from build123d import *

# Parameters (mm, degrees)
SKETCH_1_R               = 23.15
EXTRUDE_1_DEPTH          = 19
SKETCH_2_R               = 3.3
CUT_EXTRUDE_1_DEPTH      = 1
CUT_EXTRUDE_1_DEPTH_BACK = 20
PATTERN_CIRCULAR_1_COUNT = 4
FILLET_1_R               = 1
SKETCH_6_R               = 23.65
EXTRUDE_2_DEPTH          = 0.5
SKETCH_7_R               = 23.65
SKETCH_7_R_2             = 23.15
EXTRUDE_1_2_DEPTH        = 3.5
EXTRUDE_5_DEPTH          = 6
PATTERN_CIRCULAR_3_COUNT = 8
SKETCH_18_R              = 3.3
CUT_EXTRUDE_2_DEPTH      = 7.5
SKETCH_19_R              = 6.3
SKETCH_19_R_2            = 3.3
EXTRUDE_6_DEPTH          = 4
CHAMFER_1_SIZE           = 1
FILLET_3_R               = 0.5
FILLET_4_R               = 0.5


with BuildPart() as part:
    # Sketch 1 → Extrude 1 (new body)
    with BuildSketch(Plane(origin=(0, 0, 0), x_dir=(1, 0, 0), z_dir=(0, 1, 0))):
        Circle(SKETCH_1_R)
    extrude(amount=EXTRUDE_1_DEPTH)

    # Sketch 5 → Hole Wizard M3 _1 (revolve, cut)
    with BuildSketch(Plane(origin=(-12, 19, 0), x_dir=(0, 0, 1), z_dir=(1, 0, 0))):
        Polygon((0, 0), (0, 4.751075774), (1.25, 4), (1.25, 0), align=None)
    hole_wizard_m3_1 = revolve(axis=Axis((-12, 25.35, 0), (0, -1, 0)), mode=Mode.SUBTRACT)

    # Sketch 2 → Cut-Extrude 1 (cut, two sides)
    with BuildSketch(Plane(origin=(0, 19, 0), x_dir=(1, 0, 0), z_dir=(0, 1, 0))) as cut_extrude_1_sk:
        Circle(SKETCH_2_R)
    extrude(amount=CUT_EXTRUDE_1_DEPTH, mode=Mode.SUBTRACT)
    extrude(cut_extrude_1_sk.sketch, amount=-CUT_EXTRUDE_1_DEPTH_BACK, mode=Mode.SUBTRACT)

    # Pattern Circular 1: Hole Wizard M3 _1 ×4 about axis
    pattern_circular_1_axis = Axis((0, 0, 0), (0, 1, 0))
    for i in range(1, PATTERN_CIRCULAR_1_COUNT):
        add(hole_wizard_m3_1.rotate(pattern_circular_1_axis, i * 360 / PATTERN_CIRCULAR_1_COUNT), mode=Mode.SUBTRACT)

    # Fillet 1
    fillet_1_edges = [part.edges().sort_by_distance(p)[0] for p in [
        (-23.15, 19, 0),
    ]]
    fillet(fillet_1_edges, radius=FILLET_1_R)

    # Sketch 6 → Extrude 2 (add)
    with BuildSketch(Plane.XZ):
        Circle(SKETCH_6_R)
    extrude(amount=EXTRUDE_2_DEPTH)

    # Sketch 7 → Extrude 1 2 (add)
    with BuildSketch(Plane.XZ.offset(0.5)):
        Circle(SKETCH_7_R)
        Circle(SKETCH_7_R_2, mode=Mode.SUBTRACT)
    extrude(amount=EXTRUDE_1_2_DEPTH)

    # Sketch 8 → Extrude 5 (add)
    with BuildSketch(Plane.XZ.offset(0.5)):
        with BuildLine():
            Line((-21.839675903, 3.694733612), (-22.825665785, 3.861538741))
            ThreePointArc((-22.825665785, 3.861538741), (-23.15, 0), (-22.825665785, -3.861538741))
            Line((-22.825665785, -3.861538741), (-21.839675903, -3.694733612))
            ThreePointArc((-21.839675903, -3.694733612), (-20.969056247, -2.594652523), (-19.772134146, -1.862850316))
            ThreePointArc((-19.772134146, -1.862850316), (-18.5, 0), (-19.772134146, 1.862850316))
            ThreePointArc((-19.772134146, 1.862850316), (-20.969056247, 2.594652523), (-21.839675903, 3.694733612))
        make_face()
        with BuildLine():
            ThreePointArc((-13.409662832, 18.870703292), (-16.369521984, 16.369521984), (-18.870703292, 13.409662832))
            Line((-18.870703292, 13.409662832), (-18.055554121, 12.830411738))
            ThreePointArc((-18.055554121, 12.830411738), (-16.662058262, 12.992665473), (-15.298244224, 12.663776043))
            ThreePointArc((-15.298244224, 12.663776043), (-13.081475452, 13.081475452), (-12.663776043, 15.298244224))
            ThreePointArc((-12.663776043, 15.298244224), (-12.992665473, 16.662058262), (-12.830411738, 18.055554121))
            Line((-12.830411738, 18.055554121), (-13.409662832, 18.870703292))
        make_face()
        with BuildLine():
            Line((-18.055554121, -12.830411738), (-18.870703292, -13.409662832))
            ThreePointArc((-18.870703292, -13.409662832), (-16.369521984, -16.369521984), (-13.409662832, -18.870703292))
            Line((-13.409662832, -18.870703292), (-12.830411738, -18.055554121))
            ThreePointArc((-12.830411738, -18.055554121), (-12.992665473, -16.662058261), (-12.663776043, -15.298244224))
            ThreePointArc((-12.663776043, -15.298244224), (-13.081475452, -13.081475452), (-15.298244224, -12.663776043))
            ThreePointArc((-15.298244224, -12.663776043), (-16.662058261, -12.992665473), (-18.055554121, -12.830411738))
        make_face()
        with BuildLine():
            ThreePointArc((18.870703292, 13.409662832), (16.369521984, 16.369521984), (13.409662832, 18.870703292))
            Line((13.409662832, 18.870703292), (12.830411738, 18.055554121))
            ThreePointArc((12.830411738, 18.055554121), (12.992665473, 16.662058262), (12.663776043, 15.298244224))
            ThreePointArc((12.663776043, 15.298244224), (13.081475452, 13.081475452), (15.298244224, 12.663776043))
            ThreePointArc((15.298244224, 12.663776043), (16.662058261, 12.992665473), (18.055554121, 12.830411738))
            Line((18.055554121, 12.830411738), (18.870703292, 13.409662832))
        make_face()
        with BuildLine():
            Line((12.830411738, -18.055554121), (13.409662832, -18.870703292))
            ThreePointArc((13.409662832, -18.870703292), (16.369521984, -16.369521984), (18.870703292, -13.409662832))
            Line((18.870703292, -13.409662832), (18.055554121, -12.830411738))
            ThreePointArc((18.055554121, -12.830411738), (16.662058262, -12.992665473), (15.298244224, -12.663776043))
            ThreePointArc((15.298244224, -12.663776043), (13.081475452, -13.081475452), (12.663776043, -15.298244224))
            ThreePointArc((12.663776043, -15.298244224), (12.992665473, -16.662058261), (12.830411738, -18.055554121))
        make_face()
        with BuildLine():
            ThreePointArc((22.825665785, -3.861538741), (23.15, 0), (22.825665785, 3.861538741))
            Line((22.825665785, 3.861538741), (21.839675903, 3.694733612))
            ThreePointArc((21.839675903, 3.694733612), (20.969056247, 2.594652523), (19.772134146, 1.862850316))
            ThreePointArc((19.772134146, 1.862850316), (18.5, 0), (19.772134146, -1.862850316))
            ThreePointArc((19.772134146, -1.862850316), (20.969056247, -2.594652523), (21.839675903, -3.694733612))
            Line((21.839675903, -3.694733612), (22.825665785, -3.861538741))
        make_face()
    extrude(amount=EXTRUDE_5_DEPTH)

    # Sketch 17 → Hole Wizard M2 _1 (revolve, cut)
    with BuildSketch(Plane(origin=(-20.5, -6.5, 0), x_dir=(0, 0, -1), z_dir=(1, 0, 0))):
        Polygon((0, 0), (0, 5.680688495), (0.8, 5.2), (0.8, 0), align=None)
    hole_wizard_m2_1 = revolve(axis=Axis((-20.5, -12.85, 0), (0, 1, 0)), mode=Mode.SUBTRACT)

    # Pattern Circular 3: Hole Wizard M2 _1 ×8 about axis, 1 skipped
    pattern_circular_3_axis = Axis((0, 0, 0), (0, 1, 0))
    add([hole_wizard_m2_1.rotate(pattern_circular_3_axis, i * 360 / PATTERN_CIRCULAR_3_COUNT) for i in range(1, PATTERN_CIRCULAR_3_COUNT) if i not in (2,)], mode=Mode.SUBTRACT)

    # Sketch 18 → Cut-Extrude 2 (cut, through all)
    with BuildSketch(Plane(origin=(0, 0, 0), x_dir=(1, 0, 0), z_dir=(0, 1, 0))):
        Circle(SKETCH_18_R)
    extrude(amount=-CUT_EXTRUDE_2_DEPTH, mode=Mode.SUBTRACT)

    # Sketch 19 → Extrude 6 (add)
    with BuildSketch(Plane.XZ.offset(0.5)):
        Circle(SKETCH_19_R)
        Circle(SKETCH_19_R_2, mode=Mode.SUBTRACT)
    extrude(amount=EXTRUDE_6_DEPTH)

    # Chamfer 1
    chamfer_1_edges = [part.edges().sort_by_distance(p)[0] for p in [
        (-3.3, 19, 0),
    ]]
    chamfer(chamfer_1_edges, length=CHAMFER_1_SIZE)

    # Fillet 3
    fillet_3_edges = [part.edges().sort_by_distance(p)[0] for p in [
        (-6.3, -4.5, 0),
    ]]
    fillet(fillet_3_edges, radius=FILLET_3_R)

    # Fillet 4
    fillet_4_edges = [part.edges().sort_by_distance(p)[0] for p in [
        (-3.3, -4.5, 0),
    ]]
    fillet(fillet_4_edges, radius=FILLET_4_R)


solid = part.part
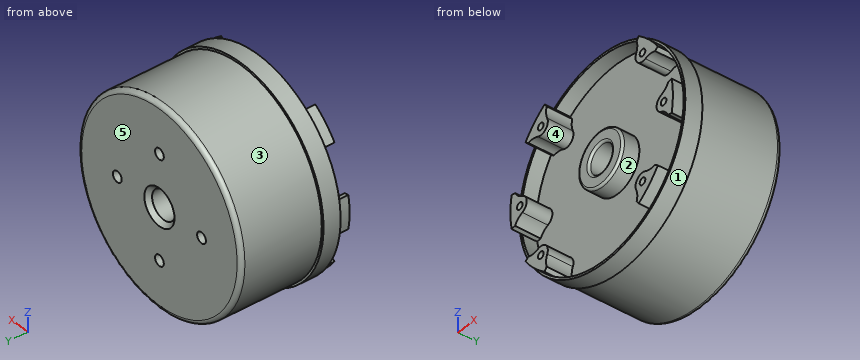
CAD build for the part. Positions are in the model's coordinates, mm. Face numbers are marked on the shaded views. A direction names the side the tool comes from. Coordinates: 2 decimals unless noted, no trailing zeros. Write each loop counter-clockwise with the first axis right and the second up, starting at its lowest first coordinate (ties: lowest second). Pieces come first, ordered by that corner, then holes. Notation, with made-up numbers: M 17.5,53 L 70.5,53 A12 cw 70.5,60 Z; hole C -20,-25.5 d1. An arc over 180 degrees is marked long. Return JSON: item names as keys, results as strings.
Item 1: Drop flat-ended pins along their axis: pin 1 Ø3 at (y, z) = (14, -14.5) entering from +X; pin 2 Ø1 at (y, z) = (15, -3) entering from +X; pin 3 Ø8.5 at (x, z) = (0, 0) entering from +Y. Give the stop position or say it passes through.
Findings below:
{"pin 1": "stops at x = 19.16", "pin 2": "stops at x = 23.01", "pin 3": "stops at y = 18.95"}
Item 2: Slice it at A-A, the plane y = 10. Write the cut outline in (x, z).
Findings below:
{"outline": "C 0,0 d46.3; hole C 0,0 d6.6"}
Item 3: Probe line 1 (Z direction, x = 0, y = 16.1); line 2 (Y direction, x = -12, z = 17); line 3 (Z direction, x = 20.5, y = 15.25). List the from-to ranges inside material, lowest first. Write a range as from..to.
Findings below:
{"line 1": "z = -23.15..-13.25, -10.75..-3.3, 3.3..10.75, 13.25..23.15", "line 2": "y = -0.5..19", "line 3": "z = -10.76..10.76"}
Item 4: Two-plate mould, pull along X, no slides. Class the marked faces 3, 4 and 5: +X half, -X half, draft (parallel to the pull), parting line (faces both ways), or undercut.
Findings below:
{"face 3": "parting line", "face 4": "undercut", "face 5": "draft"}
Item 5: Which spindle directions (+Z, -Z, +X, -X, +Y, -Y) get a long thin tool onto all of the face, cutting with end or side? Do the marked faces 1 and 2. Say none if no direction does.
Findings below:
{"face 1": "+Y, -Y", "face 2": "-Y"}
